from build123d import *

# Parameters (mm, degrees)
SKETCH_R             = 7.5
PAD_DEPTH            = 40
SKETCH001_R          = 5.25
POCKET_DEPTH         = 30
SKETCH002_R          = 5.25
POCKET001_DEPTH      = 30
SKETCH004_W          = 18
SKETCH004_H          = 18
PAD001_DEPTH         = 9
SKETCH005_R          = 3.5
POCKET002_DEPTH      = 40.001
POCKET002_DEPTH_BACK = 40.001
SKETCH006_R          = 3
POCKET003_DEPTH      = 9.001
POCKET003_DEPTH_BACK = 9.001
SKETCH008_W          = 13
SKETCH008_H          = 13
POCKET004_DEPTH      = 16.5
FILLET_R             = 1


with BuildPart() as part:
    # Sketch → Pad (new body, symmetric)
    with BuildSketch(Plane.XZ):
        Circle(SKETCH_R)
    extrude(amount=PAD_DEPTH, both=True)

    # Sketch001 → Pocket (cut)
    with BuildSketch(Plane.XZ.offset(40)):
        Circle(SKETCH001_R)
    extrude(amount=-POCKET_DEPTH, mode=Mode.SUBTRACT)

    # Sketch002 → Pocket001 (cut)
    with BuildSketch(Plane.XZ.offset(-40)):
        Circle(SKETCH002_R)
    extrude(amount=POCKET001_DEPTH, mode=Mode.SUBTRACT)

    # Sketch004 → Pad001 (join, symmetric)
    with BuildSketch(Plane.YZ):
        Rectangle(SKETCH004_W, SKETCH004_H)
    extrude(amount=PAD001_DEPTH, both=True)

    # Sketch005 → Pocket002 (cut, two sides)
    with BuildSketch(Plane.XZ) as pocket002_sk:
        Circle(SKETCH005_R)
    extrude(amount=-POCKET002_DEPTH, mode=Mode.SUBTRACT)
    extrude(pocket002_sk.sketch, amount=POCKET002_DEPTH_BACK, mode=Mode.SUBTRACT)

    # Sketch006 → Pocket003 (cut, two sides)
    with BuildSketch(Plane.XY) as pocket003_sk:
        Circle(SKETCH006_R)
    extrude(amount=-POCKET003_DEPTH, mode=Mode.SUBTRACT)
    extrude(pocket003_sk.sketch, amount=POCKET003_DEPTH_BACK, mode=Mode.SUBTRACT)

    # Sketch008 → Pocket004 (cut)
    with BuildSketch(Plane.XY.offset(9)):
        Rectangle(SKETCH008_W, SKETCH008_H)
    extrude(amount=-POCKET004_DEPTH, mode=Mode.SUBTRACT)

    # Fillet
    fillet_edges = [part.edges().sort_by_distance(p)[0] for p in [
        (-9, 0, -9),
        (0, -9, -9),
        (0, 9, -9),
        (9, 0, -9),
        (9, 9, 0),
        (9, -9, 0),
        (9, 0, 9),
        (-9, 9, 0),
        (-9, -9, 0),
        (-9, 0, 9),
        (0, 9, 9),
        (0, -9, 9),
    ]]
    fillet(fillet_edges, radius=FILLET_R)


solid = part.part
Design review of the part built by this model. Coordinates are the model's own, in mm. A direction names the side the tool comes from. Round coordinates to 2 decimals unless told otherwise and drop trailing zeros. Loops run counter-clockwise (first coordinate to the right, second up) from the corner with the lowest first, then second, coordinate; pieces in that order, holes last. Notation, with made-up numbers: (-9.75, 52.5) - (36.25, 52.5) arc R14 ccw to (36.25, 65.5) - close; hole circle Ø10 at (12.5, 51.25). An arc over 180 degrees is marked (long way). One line per question, with ' | ' between items.
1. For faces 1 (the face through (0, 7, 9)), 2 (the face through (-3, -6.5, 3)), 3 (the face through (0, 10, 4)), 4 (the face through (5, -25.2, 1.6)), list the 3-axis set-ups (+Z, -Z, +X, -X, +Y, -Y) from which the entire face can be reached by the end or side of a thin tool; tool diameter is ignored.
Results are:
face 1: +Z, +X, -X, +Y, -Y | face 2: +Z | face 3: +Y | face 4: -Y
2. For L1, parallel to Z at x = 0, y = 19.25; L2, parallel to Y at x = 3.5, z = 7, list the stretches that pass through material, from the lowest coordinate up. Write a range as [from, to].
Results are:
L1: z = [-7.5, -5.25], [5.25, 7.5] | L2: y = [-9, -6.5], [6.5, 9]
3. We need section B-B, the plane x = 0. State how many separate pieces and enclosed holes the cut face has, and give its area (3 significant figures).
Results are:
separate pieces: 4 | enclosed holes: 0 | area: 351 mm²
4. We need section A-A, the plane y = 0. State the section outline as (x, z) points, and give its area (3 significant figures).
Results are:
outline: (-9, -8) arc R1 ccw to (-8, -9) - (-3, -9) - (-3, -7.5) - (-6.5, -7.5) - (-6.5, 9) - (-8, 9) arc R1 ccw to (-9, 8) - close; (3, -9) - (8, -9) arc R1 ccw to (9, -8) - (9, 8) arc R1 ccw to (8, 9) - (6.5, 9) - (6.5, -7.5) - (3, -7.5) - close | area: 99.6 mm²
5. Clearance check with flat-ended pins moving along their axes: P1, Ø9.5, axis at x = 0, z = 0, coming from the +Y side; P2, Ø3, axis at x = 3.5, z = -0.5, coming from the -Y side; P3, Ø4, axis at x = -2.5, y = 20.5, coming from the +Z side. State where each tip first meets the part, or that it passes through.
Results are:
P1: stops at y = 10 | P2: stops at y = -10 | P3: stops at z = 7.48
6. Draft analysis for pull direction Z (two halves, no side actions). For faces 5 (the face through (0, -10, 4)), 6 (the face through (-7.493, -24.717, 0.33)), 7 (the face through (-3, 0, -8)), state which applies: released by +Z, released by -Z, zero draft, split by the parting line, or undercut.
Results are:
face 5: undercut | face 6: split by the parting line | face 7: zero draft
7. We need section C-C, the plane z = 6.75. State the section outline as (x, y) points, and give its area (3 significant figures).
Results are:
outline: (-9, -8) arc R1 ccw to (-8, -9) - (-3.27, -9) - (-3.27, -40) - (3.27, -40) - (3.27, -9) - (8, -9) arc R1 ccw to (9, -8) - (9, 8) arc R1 ccw to (8, 9) - (3.27, 9) - (3.27, 40) - (-3.27, 40) - (-3.27, 9) - (-8, 9) arc R1 ccw to (-9, 8) - close; hole (-6.5, -6.5) - (6.5, -6.5) - (6.5, 6.5) - (-6.5, 6.5) - close | area: 560 mm²
8. We need section D-D, the plane y = -16. State the section outline as (x, z) points.
Results are:
outline: circle Ø15 at (0, 0); hole circle Ø10.5 at (0, 0)
